The model under review builds one solid part; all positions refer to its coordinate system, in mm. A direction names the side the tool comes from. Coordinates: 2 decimals unless noted, no trailing zeros. Write each loop counter-clockwise with the first axis right and the second up, starting at its lowest first coordinate (ties: lowest second). Pieces come first, ordered by that corner, then holes.
```python
from build123d import *

# Parameters (mm, degrees)
SKETCH1_W           = 171.681197847
SKETCH1_H           = 28.969428325
SKETCH1_R           = 1.65
BOSS_EXTRUDE1_DEPTH = 1
SKETCH7_W           = 171.681197847
SKETCH7_H           = 25.151518983
BOSS_EXTRUDE2_DEPTH = 5


with BuildPart() as part:
    # Sketch1 → Boss-Extrude1 (new body)
    with BuildSketch(Plane.XY):
        with Locations((-137.259678888, 258.015285838)):
            Rectangle(SKETCH1_W, SKETCH1_H)
        with Locations((-208.100277812, 267.5)):
            Circle(SKETCH1_R, mode=Mode.SUBTRACT)
        with Locations((-138.100277812, 267.5)):
            Circle(SKETCH1_R, mode=Mode.SUBTRACT)
        with Locations((-68.100277811, 267.5)):
            Circle(SKETCH1_R, mode=Mode.SUBTRACT)
    extrude(amount=BOSS_EXTRUDE1_DEPTH)

    # Sketch7 → Boss-Extrude2 (add)
    with BuildSketch(Plane(origin=(0, 272.5, 0), x_dir=(1, 0, 0), z_dir=(0, 1, 0))):
        with Locations((-137.259678888, 11.575759492)):
            Rectangle(SKETCH7_W, SKETCH7_H)
    extrude(amount=BOSS_EXTRUDE2_DEPTH)


solid = part.part
```
Item 1: Take a section at D-D, the plane z = -13. Write out the cut boundary in (x, y).
Solved:
outline: (-223.1, 272.5) - (-51.42, 272.5) - (-51.42, 277.5) - (-223.1, 277.5) - close
Item 2: Take a section at C-C, the plane y = 251.5. Write out the cut boundary in (x, z).
Solved:
outline: (-223.1, 0) - (-51.42, 0) - (-51.42, 1) - (-223.1, 1) - close
Item 3: To check wall thickness, follow line 1 along X through (y, z) = (267.5, 0.55); line 2 along Y through (x, z) = (-85, -19); line 3 along Z through (x, y) = (-132.5, 260). State the ranges of each line that lie inside material, in increasing order.
Solved:
line 1: x = -223.1 to -209.75, -206.45 to -139.75, -136.45 to -69.75, -66.45 to -51.42
line 2: y = 272.5 to 277.5
line 3: z = 0 to 1
Item 4: Mouldability with a two-part tool opening along Y and no side actions: class faces 1 (the face through (-68.5, 265.9, 0.5)), 2 (the face through (-138, 277.5, -12)), 3 (the face through (-138, 275, -24.152)) as pulls with the +Y half, pulls with the -Y half, needs draft (parallel to the pull), parting line crosses it, or undercut.
Solved:
face 1: undercut
face 2: pulls with the +Y half
face 3: needs draft
Item 5: Take a section at B-B, the plane x = -157.5. Write out the cut boundary in (y, z), plus the area to 3 significant figures.
Solved:
outline: (243.53, 0) - (272.5, 0) - (272.5, -24.15) - (277.5, -24.15) - (277.5, 1) - (243.53, 1) - close
area: 155 mm2
Item 6: For pin 1 (8 mm diameter, centred on x = -122.5, z = -5.5, fed in from -Y); pin 2 (8.5 mm diameter, centred on x = -178, y = 259.5, fed in from -Z), all flat-tipped, find the tip position at first contact; note any pin that passes through.
Solved:
pin 1: stops at y = 272.5
pin 2: stops at z = 0
Item 7: Take a section at A-A, the plane y = 267.5. Write out the cut boundary in (x, z), plus the area to 3 significant figures.
Solved:
outline: (-223.1, 0) - (-209.75, 0) - (-209.75, 1) - (-223.1, 1) - close; (-206.45, 0) - (-139.75, 0) - (-139.75, 1) - (-206.45, 1) - close; (-136.45, 0) - (-69.75, 0) - (-69.75, 1) - (-136.45, 1) - close; (-66.45, 0) - (-51.42, 0) - (-51.42, 1) - (-66.45, 1) - close
area: 162 mm2
Item 8: Machinability: for faces 4 (the face through (-223.1, 273, -10)), 5 (the face through (-138, 272.5, -12)), which of the approach directions +Z, -Z, +X, -X, +Y, -Y give a long, thin tool a straight path to every point of the face, cutting with its end or side? Answer none if there is none.
Solved:
face 4: +Z, -Z, -X, +Y, -Y
face 5: -Z, +X, -X, -Y
